Print and shaded views of the part. All mm, measured from the part's lowest x, y and z. A direction names the side the tool comes from. Round coordinates to 2 decimals unless told otherwise and drop trailing zeros. Write each loop counter-clockwise with the first axis right and the second up, starting at its lowest first coordinate (ties: lowest second). Pieces come first, ordered by that corner, then holes. Notation, with made-up numbers: M -28.5,34 L -8.5,34 A11 ccw -8.5,40 Z; hole C 53,64.5 d8. An arc over 180 degrees is marked long. Write item = value, one per line. Start each with the question number.
Q1. Band-saw the part on D-D on z = 3. Write the cut outline in (x, y), plus the area to 3 significant figures.
Q2. Band-saw the part on B-B on y = 14.5. Write the cut outline in (x, z).
Q3. Tool access for the marked faces 3 and 4: list every direction of +Z, -Z, +X, -X, +Y, -Y with a clear straight run to the whole face (end or side of a thin tool).
Q4. Drop flat-ended pins along their axis: P1, Ø2, axis at y = 11, z = 7.5, coming from the +X side; P2, Ø10, axis at x = 33, z = 6, coming from the -Y side; P3, Ø6, axis at x = 18.5, z = 8, coming from the +Y side. Give the stop position or say it passes through.
Q5. Band-saw the part on A-A on x = 14. Write the cut outline in (y, z).
Q6. Probe L1, parallel to Z at x = 15, y = 2; L2, parallel to Y at x = 20.5, z = 17.75; L3, parallel to Y at x = 23, z = 7. List the from-to ranges inside material, lowest first.
Q7. Pull direction X, two halves, no side cores. Call the marked faces 1 and 2: released by +X, released by -X, zero draft, split by the parting line, or undercut.
Q8. Band-saw the part on C-C on z = 14.25. Write the cut outline in (x, y), plus the area to 3 significant figures.
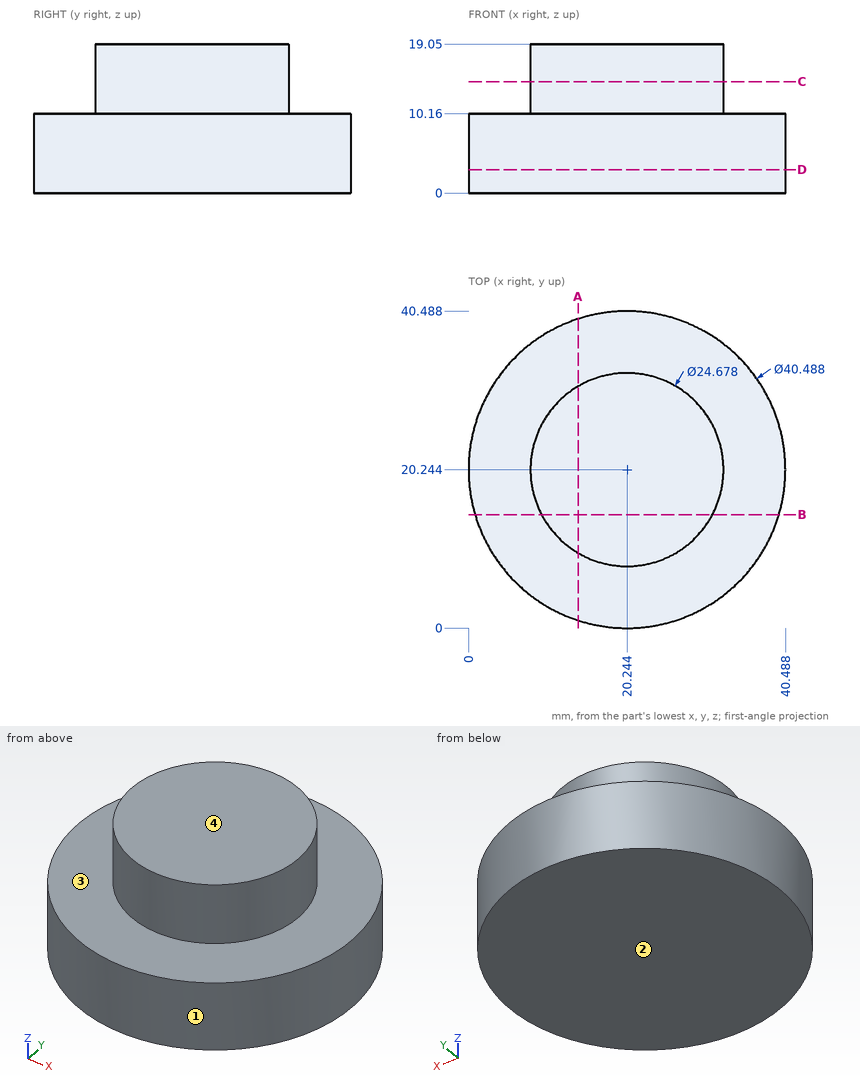
Conclusion:
q1.outline = C 20.24,20.24 d40.49
q1.area = 1,290 mm^2
q2.outline = M 0.83,0 L 39.66,0 L 39.66,10.16 L 31.16,10.16 L 31.16,19.05 L 9.32,19.05 L 9.32,10.16 L 0.83,10.16 Z
q3.face_3 = +Z
q3.face_4 = +Z, +X, -X, +Y, -Y
q4.P1 = 38.73
q4.P2 = 1.54
q4.P3 = 40.49
q5.outline = M 0.99,0 L 39.5,0 L 39.5,10.16 L 30.89,10.16 L 30.89,19.05 L 9.6,19.05 L 9.6,10.16 L 0.99,10.16 Z
q6.L1 = 0 to 10.16
q6.L2 = 7.91 to 32.58
q6.L3 = 0.19 to 40.3
q7.face_1 = split by the parting line
q7.face_2 = zero draft
q8.outline = C 20.24,20.24 d24.68
q8.area = 478 mm^2
